Read the model definition and answer for the solid it produces. Units are mm, in the model's axes. A direction names the side the tool comes from. Give positions to 0.01 mm unless a question says otherwise; leave off trailing zeros. Write each loop counter-clockwise with the first axis right and the second up, starting at its lowest first coordinate (ties: lowest second). Pieces come first, ordered by that corner, then holes. Notation, with made-up numbers: (-25, 4) -> (19, 4) arc R29 cw to (19, 35) -> close; hole circle Ø3 at (27, 1.5). An arc over 180 degrees is marked (long way). Write item = value, one per line.
from build123d import *

# Parameters (mm, degrees)
SKETCH_1_R          = 2.95
SKETCH_1_R_2        = 1.5
EXTRUDE_1_DEPTH     = 20
CUT_EXTRUDE_1_DEPTH = 3


with BuildPart() as part:
    # Эскиз1 → Бобышка-Вытянуть1 (new body)
    with BuildSketch(Plane(origin=(0, 0, 0), x_dir=(0, 0, -1), z_dir=(1, 0, 0))):
        with BuildLine():
            Line((-4.215373649, -1.575), (-2.576061674, -5.9625))
            ThreePointArc((-2.576061674, -5.9625), (0, -7.75), (2.576061674, -5.9625))
            Line((2.576061674, -5.9625), (4.215373649, -1.575))
            ThreePointArc((4.215373649, -1.575), (0, 4.5), (-4.215373649, -1.575))
        make_face()
        Circle(SKETCH_1_R, mode=Mode.SUBTRACT)
        with Locations((0, -5)):
            Circle(SKETCH_1_R_2, mode=Mode.SUBTRACT)
    extrude(amount=EXTRUDE_1_DEPTH)

    # Эскиз2 → Вырез-Вытянуть1 (cut)
    with BuildSketch(Plane(origin=(20, 0, 0), x_dir=(0, 0, -1), z_dir=(1, 0, 0))):
        with BuildLine():
            Line((-1.5, -5), (1.5, -5))
            Line((1.5, -5), (1.5, -3.272613634))
            ThreePointArc((1.5, -3.272613634), (0, 3.6), (-1.5, -3.272613634))
            Line((-1.5, -3.272613634), (-1.5, -5))
        make_face()
    extrude(amount=-CUT_EXTRUDE_1_DEPTH, mode=Mode.SUBTRACT)


solid = part.part
(1) The part is cut by section D-D on z = 3.25. Determine the outline of the cut face in (x, y).
Checks:
outline = (0, -4.16) -> (20, -4.16) -> (20, -1.55) -> (17, -1.55) -> (17, 1.55) -> (20, 1.55) -> (20, 3.11) -> (0, 3.11) -> close
(2) A tool of negligible diameter and unlimited length cuts with its end or side. For faces 5 (the flat face through (19, -4, 1.5)), 6 (the cylindrical face through (9.9, 4.5, -0.1)), from which of +Z, -Z, +X, -X, +Y, -Y can it reach the whole face along a straight path? Write none if from no direction.
Checks:
face_5 = +X
face_6 = +X, -X
(3) Consider L1, parallel to Y at x = 12.5, z = 0; L2, parallel to Z at x = 10.75, y = 0; L3, parallel to Y at x = 12.75, z = -1.25. Determine where each line is inside the solid, lowest interval first.
Checks:
L1 = -7.75 to -6.5, -3.5 to -2.95, 2.95 to 4.5
L2 = -4.5 to -2.95, 2.95 to 4.5
L3 = -7.45 to -5.83, -4.17 to -2.67, 2.67 to 4.32
(4) The part is cut by section C-C on x = 14. Count the separate pieces of the cut face and the enclosed holes in it, plus the area to 3 significant figures.
Checks:
separate_pieces = 1
enclosed_holes = 2
area = 47.8 mm²
(5) The part is cut by section A-A on z = 0. Determine the outline of the cut face in (x, y), plus the area to 3 significant figures.
Checks:
outline = (0, -7.75) -> (20, -7.75) -> (20, -6.5) -> (0, -6.5) -> close; (0, -3.5) -> (17, -3.5) -> (17, -2.95) -> (0, -2.95) -> close; (0, 2.95) -> (17, 2.95) -> (17, 3.6) -> (20, 3.6) -> (20, 4.5) -> (0, 4.5) -> close
area = 63.4 mm²
(6) The part is cut by section B-B on y = 0. Determine the outline of the cut face in (x, z), plus the area to 3 significant figures.
Checks:
outline = (0, -4.5) -> (20, -4.5) -> (20, -3.6) -> (17, -3.6) -> (17, -2.95) -> (0, -2.95) -> close; (0, 2.95) -> (17, 2.95) -> (17, 3.6) -> (20, 3.6) -> (20, 4.5) -> (0, 4.5) -> close
area = 58.1 mm²
(7) For a pull along Y with two mould halves and no side action, classify faces 1 (the flat face through (9.86, -3.738, 3.407)), 2 (the cylindrical face through (9.86, -6.464, 0.325)), 3 (the flat face through (0, -3, 1)), 4 (the flat face through (17, -3, 1)) as released by +Y, released by -Y, zero draft, split by the parting line, or undercut.
Checks:
face_1 = released by -Y
face_2 = undercut
face_3 = zero draft
face_4 = undercut
(8) Given P1, Ø1.9, axis at x = 18.5, y = -4, coming from the -Z side; P2, Ø6, axis at x = 3.5, y = 1, coming from the +Z side; P3, Ø2, axis at x = 2.5, y = -3.5, coming from the -Z side; P4, Ø1.5, axis at x = 6.5, y = -6.5, coming from the -Z side, each flat-ended and moving along its own axis, determine where each tip first touches the part or whether it passes through.
Checks:
P1 = -3.66
P2 = 4.5
P3 = -3.87
P4 = -2.66
